Geometry: final body of the model. Coordinates: model frame, mm. Face numbers are marked on the shaded views. A direction names the side the tool comes from. Give positions to 0.01 mm unless a question says otherwise; leave off trailing zeros. Write each loop counter-clockwise with the first axis right and the second up, starting at its lowest first coordinate (ties: lowest second). Pieces come first, ordered by that corner, then holes.
Autodesk Inventor part; units mm, degrees
ref_plane "YZ Plane" through (0, 0, 0) normal (1, 0, 0) x (0, 1, 0)
ref_plane "XZ Plane" through (0, 0, 0) normal (0, 1, 0) x (-1, 0, 0)
ref_plane "XY Plane" through (0, 0, 0) normal (0, 0, 1) x (1, 0, 0)
sketch "Sketch1" plane through (0, 0, 0) normal (0, 0, 1) x (1, 0, 0)
  line L0 (-150, 322) -> (0, 322)
  line L1 (0, 322) -> (0, 0)
  line L2 (0, 0) -> (-150, 0)
  line L3 (-150, 0) -> (-150, 322)
  dimension "d0" = 150
  dimension "d1" = 322
extrude "Extrusion1" add sketch "Sketch1" along normal blind 150
sketch "Sketch2" plane through (0, 0, 150) normal (0, 0, 1) x (1, 0, 0)
  line L0 (0, 0) -> (0, 322)
  line L1 (0, 322) -> (-150, 322)
  point P0 (-75, 247)
  dimension "d4" = 75
  dimension "d5" = 75
hole "Hole1" at (-75, 247, 150) direction (0, 0, -1) diameter 63.5 end through all
sketch "Sketch3" plane through (-150, 0, 0) normal (-1, 0, 0) x (0, 0, 1)
  line L0 (0, 0) -> (0, 322)
  line L1 (150, 322) -> (150, 0)
  line L2 (0, 322) -> (150, 322)
  line L3 (150, 322) -> (150, 172)
  line L4 (150, 172) -> (0, 172)
  line L5 (0, 172) -> (0, 322)
  dimension "d13" = 150
extrude "Extrusion2" add sketch "Sketch3" along normal blind 200
sketch "Sketch4" plane through (-150, 0, 0) normal (0, -1, 0) x (1, 0, 0)
  line L0 (150, 0) -> (0, 0)
  line L1 (0, 150) -> (150, 150)
  line L2 (0, 0) -> (150, 0)
  line L3 (150, 0) -> (150, 150)
  line L4 (150, 150) -> (0, 150)
  line L5 (0, 150) -> (0, 0)
extrude "Extrusion3" cut sketch "Sketch4" against normal blind 172
sketch "Sketch5" plane through (-350, 172, 150) normal (0, -1, 0) x (1, 0, 0)
  line L0 (0, -150) -> (0, 0)
  line L1 (0, -150) -> (350, -150)
  line L2 (0, 0) -> (130, 0)
  line L3 (130, 0) -> (130, -150)
  line L4 (130, -150) -> (0, -150)
  line L5 (0, -150) -> (0, 0)
  dimension "d18" = 130
extrude "Extrusion4" add sketch "Sketch5" along normal blind 172
properties part number "stand"
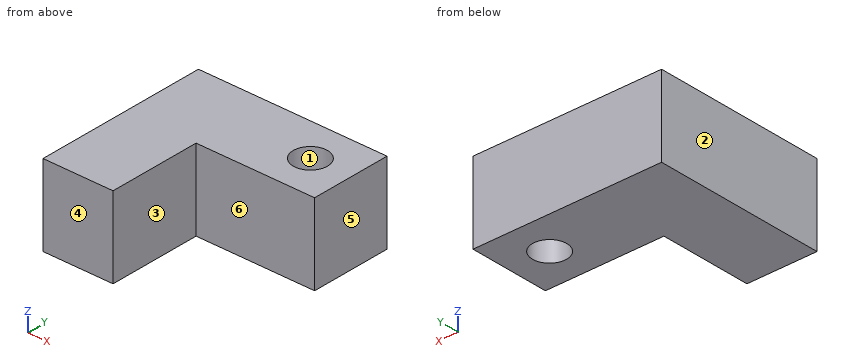
Item 1: Section D-D, the plane x = -132.5. Return the cut outline in (y, z).
Found:
outline: (172, 0) - (322, 0) - (322, 150) - (172, 150) - close
Item 2: Pull-direction query (X, two-part tool) for the marked faces 1, 2, 3 and 4; classes: +X half, -X half, draft (parallel to the pull), parting line (faces both ways), or undercut.
Found:
face 1: undercut
face 2: -X half
face 3: +X half
face 4: draft
Item 3: Section B-B, the plane x = -75. Return the cut outline in (y, z), plus the area to 3 significant figures.
Found:
outline: (172, 0) - (215.25, 0) - (215.25, 150) - (172, 150) - close; (278.75, 0) - (322, 0) - (322, 150) - (278.75, 150) - close
area: 13,000 mm2
Item 4: Line query: L1, parallel to X at y = 247, z = 37; L2, parallel to Y at x = -75, z = 100.5; L3, parallel to Y at x = -98, z = 64. Output: solid intervals per line, ascending.
Found:
L1: x = -350 to -106.75, -43.25 to 0
L2: y = 172 to 215.25, 278.75 to 322
L3: y = 172 to 225.11, 268.89 to 322
Item 5: Pin query (flat end, axial travel): pin 1 Ø10 at (y, z) = (48.5, 98) entering from +X. Return the tip coordinate at first contact, or that it passes through.
Found:
pin 1: stops at x = -220
Item 6: Section A-A, the plane y = 247. Return the cut outline in (x, z).
Found:
outline: (-350, 0) - (-106.75, 0) - (-106.75, 150) - (-350, 150) - close; (-43.25, 0) - (0, 0) - (0, 150) - (-43.25, 150) - close
Item 7: Reachability of the marked faces 5 and 6 from +Z, -Z, +X, -X, +Y, -Y: full face, straight path, thin tool, end or side. Return the list, or none.
Found:
face 5: +Z, -Z, +X, +Y, -Y
face 6: +Z, -Z, +X, -Y
Item 8: Section C-C, the plane z = 70.5. Return the cut outline in (x, y).
Found:
outline: (-350, 0) - (-220, 0) - (-220, 172) - (0, 172) - (0, 322) - (-350, 322) - close; hole circle Ø63.5 at (-75, 247)
